Could you check a few things on this drawing? It's one solid part, dimensions in mm from its lowest x, y, z. A direction names the side the tool comes from. Give positions to 0.01 mm unless a question says otherwise; leave off trailing zeros. Write each loop counter-clockwise with the first axis right and the second up, starting at its lowest first coordinate (ties: lowest second). Pieces come first, ordered by that corner, then holes.
1. Thinking about a two-plate mould opening in Y: for the marked faces 4, 5, 6 and 7, which applies, pulls with the +Y half, pulls with the -Y half, needs draft (parallel to the pull), parting line crosses it, or undercut?
2. I'm going to push flat-ended pins straight in: pin 1 (1.5 mm diameter, centred on x = 39.5, z = 23.5, fed in from +Y); pin 2 (11 mm diameter, centred on y = 55.5, z = 5, fed in from -X); pin 3 (15 mm diameter, centred on y = 20.5, z = 19.5, fed in from -X). Where does each tip first touch, or does it pass through?
3. On a 3-axis mill with a long thin cutter (end or side, diameter ignored), from which of +Z, -Z, +X, -X, +Y, -Y can I reach the whole of each face in a straight line? I mean the marked faces 1, 2 and 3. Say none if no direction works.
4. Suppose I cut it at D-D (z = 3). Please give me the cut outline in (x, y).
5. If I drill on probe 1 along Z at (x, y) = (15, 38.5); probe 2 along X at (y, z) = (65, 6.5); probe 3 along Y at (x, z) = (45, 23.5), over which ranges is the centre line in solid material (lowest first)?
6. Suppose I cut it at C-C (z = 11). Please give me the cut outline in (x, y), and give its area (4 significant figures).
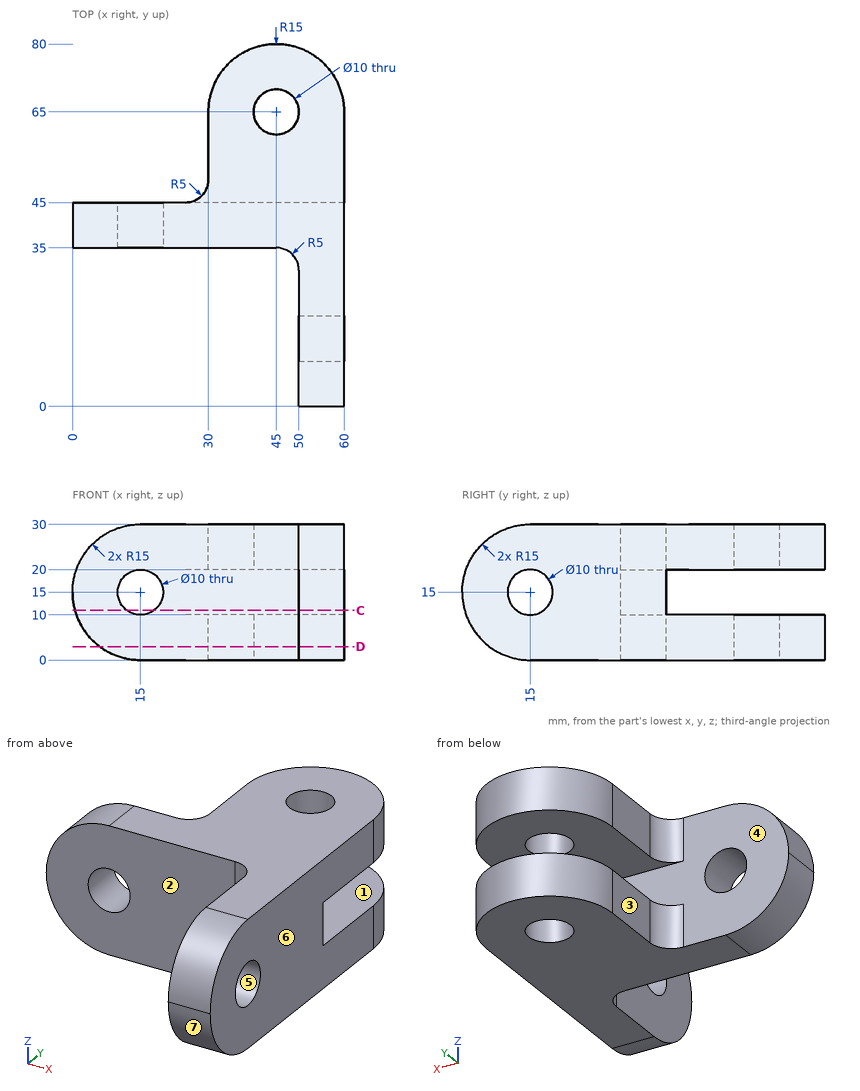
Checks:
1. face 4: pulls with the +Y half
1. face 5: undercut
1. face 6: needs draft
1. face 7: pulls with the -Y half
2. pin 1: stops at y = 79.23
2. pin 2: stops at x = 30
2. pin 3: stops at x = 50
3. face 1: +X, -X, +Y
3. face 2: +Z, -Z, -X, -Y
3. face 3: +Z, -Z, -X, +Y
4. outline: (6, 35) - (45, 35) arc R5 cw to (50, 30) - (50, 6) - (60, 6) - (60, 65) arc R15 ccw to (30, 65) - (30, 50) arc R5 cw to (25, 45) - (6, 45) - close; hole circle Ø10 at (45, 65)
5. probe 1: z = 0 to 10, 20 to 30
5. probe 2: x = 30 to 40, 50 to 60
5. probe 3: y = 35 to 60, 70 to 80
6. outline: (0.54, 35) - (12, 35) - (12, 45) - (0.54, 45) - close; (18, 35) - (45, 35) arc R5 cw to (50, 30) - (50, 18) - (60, 18) - (60, 45) - (18, 45) - close; (50, 0.54) - (60, 0.54) - (60, 12) - (50, 12) - close
6. area: 824.5 mm2
